```python
from build123d import *

# Parameters (mm, degrees)
BOSS_EXTRUDE1_DEPTH = 3.2
CUT_EXTRUDE1_DEPTH  = 1.2
SKETCH3_R           = 3.72
CUT_EXTRUDE2_DEPTH  = 26.690465157
SKETCH4_R           = 1.8
CUT_EXTRUDE3_DEPTH  = 26.811625288
SKETCH5_R           = 0.76
CUT_EXTRUDE4_DEPTH  = 10


with BuildPart() as part:
    # Sketch1 → Boss-Extrude1 (new body)
    with BuildSketch(Plane(origin=(0, 0, 0), x_dir=(1, 0, 0), z_dir=(0, 1, 0))):
        with BuildLine():
            Line((2, 0), (14, 0))
            ThreePointArc((14, 0), (15.414213562, -0.585786438), (16, -2))
            Line((16, -2), (16, -18))
            ThreePointArc((16, -18), (15.414213562, -19.414213562), (14, -20))
            Line((14, -20), (2, -20))
            ThreePointArc((2, -20), (0.585786438, -19.414213562), (0, -18))
            Line((0, -18), (0, -2))
            ThreePointArc((0, -2), (0.585786438, -0.585786438), (2, 0))
        make_face()
    extrude(amount=BOSS_EXTRUDE1_DEPTH)

    # Sketch2 → Cut-Extrude1 (cut)
    with BuildSketch(Plane(origin=(0, 3.2, 0), x_dir=(1, 0, 0), z_dir=(0, 1, 0))):
        with BuildLine():
            Line((3.2, -5.5), (12.8, -5.5))
            ThreePointArc((12.8, -5.5), (13.648528137, -5.851471863), (14, -6.7))
            Line((14, -6.7), (14, -13.3))
            ThreePointArc((14, -13.3), (13.648528137, -14.148528137), (12.8, -14.5))
            Line((12.8, -14.5), (3.2, -14.5))
            ThreePointArc((3.2, -14.5), (2.351471863, -14.148528137), (2, -13.3))
            Line((2, -13.3), (2, -6.7))
            ThreePointArc((2, -6.7), (2.351471863, -5.851471863), (3.2, -5.5))
        make_face()
    extrude(amount=-CUT_EXTRUDE1_DEPTH, mode=Mode.SUBTRACT)

    # Sketch3 → Cut-Extrude2 (cut, through all)
    with BuildSketch(Plane(origin=(0, 2, 0), x_dir=(1, 0, 0), z_dir=(0, 1, 0))):
        with Locations(Location((9.5, -10.0173545, 0), (0, 0, 270))):
            Circle(SKETCH3_R)
    extrude(amount=-CUT_EXTRUDE2_DEPTH, mode=Mode.SUBTRACT)

    # Sketch4 → Cut-Extrude3 (cut, through all)
    with BuildSketch(Plane(origin=(0, 3.2, 0), x_dir=(1, 0, 0), z_dir=(0, 1, 0))):
        with Locations(Location((8, -3, 0), (0, 0, 270))):
            Circle(SKETCH4_R)
        with Locations(Location((8, -16.936566923, 0), (0, 0, 90))):
            Circle(SKETCH4_R)
    extrude(amount=-CUT_EXTRUDE3_DEPTH, mode=Mode.SUBTRACT)

    # Sketch5 → Cut-Extrude4 (cut)
    with BuildSketch(Plane(origin=(0, 2, 0), x_dir=(1, 0, 0), z_dir=(0, 1, 0))):
        with Locations(Location((4.286808808, -10.283883288, 0), (0, 0, 270))):
            Circle(SKETCH5_R)
    extrude(amount=-CUT_EXTRUDE4_DEPTH, mode=Mode.SUBTRACT)


solid = part.part
```
Here's how the part is built. I have some questions about the finished solid (model axes, mm). A direction names the side the tool comes from. Coordinates: 2 decimals unless noted, no trailing zeros. Loops run counter-clockwise (first coordinate to the right, second up) from the corner with the lowest first, then second, coordinate; pieces in that order, holes last. Notation, with made-up numbers: (29.25, 16.5) -> (51.25, 16.5) arc R20 cw to (51.25, 27.5) -> close; hole circle Ø2 at (37, -7). An arc over 180 degrees is marked (long way). Return JSON: item names as keys, results as strings.
1) If we section it at D-D, the plane x = 11.75: Write out the boundary of the cut face in (y, z), then the cut area to 3 significant figures.
Results below:
{"outline": "(0, 0) -> (3.2, 0) -> (3.2, 5.5) -> (2, 5.5) -> (2, 7.05) -> (0, 7.05) -> close; (0, 12.98) -> (2, 12.98) -> (2, 14.5) -> (3.2, 14.5) -> (3.2, 20) -> (0, 20) -> close", "area": "41.4 mm²"}
2) Thinking about a two-plate mould opening in Z: for faces 1 (the face through (2, 3, 10)), 2 (the face through (15.4, 1.58, 0.57)), 3 (the face through (0.6, 1.58, 19.43)), 4 (the face through (16, 2, 10)), which applies, +Z half, -Z half, draft (parallel to the pull), parting line (faces both ways), or undercut?
Results below:
{"face 1": "undercut", "face 2": "-Z half", "face 3": "+Z half", "face 4": "draft"}
3) If we section it at A-A, the plane z = 3: Write out the boundary of the cut face in (x, y), then the cut area to 3 significant figures.
Results below:
{"outline": "(0, 0) -> (6.2, 0) -> (6.2, 3.2) -> (0, 3.2) -> close; (9.8, 0) -> (16, 0) -> (16, 3.2) -> (9.8, 3.2) -> close", "area": "39.7 mm²"}
4) If we section it at B-B, the plane x = 8: Write out the boundary of the cut face in (y, z).
Results below:
{"outline": "(0, 0) -> (3.2, 0) -> (3.2, 1.2) -> (0, 1.2) -> close; (0, 4.8) -> (3.2, 4.8) -> (3.2, 5.5) -> (2, 5.5) -> (2, 6.61) -> (0, 6.61) -> close; (0, 13.42) -> (2, 13.42) -> (2, 14.5) -> (3.2, 14.5) -> (3.2, 15.14) -> (0, 15.14) -> close; (0, 18.74) -> (3.2, 18.74) -> (3.2, 20) -> (0, 20) -> close"}
5) If we section it at C-C, the plane y = 0.6: Write out the boundary of the cut face in (x, z).
Results below:
{"outline": "(0, 2) arc R2 ccw to (2, 0) -> (14, 0) arc R2 ccw to (16, 2) -> (16, 18) arc R2 ccw to (14, 20) -> (2, 20) arc R2 ccw to (0, 18) -> close; hole circle Ø1.52 at (4.29, 10.28); hole circle Ø7.44 at (9.5, 10.02); hole circle Ø3.6 at (8, 3); hole circle Ø3.6 at (8, 16.94)"}
6) Will this pin go through, and if not, where does the flat tip stop? pin 1 (2 mm diameter, centred on x = 4.29, z = 10.28, fed in from +Y).
Results below:
{"pin 1": "y = 2"}
7) I need wall thicknesses on line 1 (X direction, y = 2.75, z = 9.25); line 2 (X direction, y = 2.55, z = 3); line 3 (Z direction, x = 7.75, y = 0.75). Which ranges of each line are inside material? Lowest first, please. Write a range as from..to.
Results below:
{"line 1": "0..2, 14..16", "line 2": "0..6.2, 9.8..16", "line 3": "0..1.22, 4.78..6.73, 13.3..15.15, 18.72..20"}
8) For faces 5 (the face through (13.639, 2.608, 5.842)), 6 (the face through (6.243, 1.622, 2.61)), which set-ups out of +Z, -Z, +X, -X, +Y, -Y let a thin tool reach every point of the face, with its end or its side?
Results below:
{"face 5": "+Y", "face 6": "+Y, -Y"}
